Design review of the part built by this model. Coordinates are the model's own, in mm. A direction names the side the tool comes from. Coordinates: 2 decimals unless noted, no trailing zeros. Loops run counter-clockwise (first coordinate to the right, second up) from the corner with the lowest first, then second, coordinate; pieces in that order, holes last. Notation, with made-up numbers: M 51,63 L 84,63 A26 ccw 84,99 Z; hole C 2,17.25 d7. An arc over 180 degrees is marked long. Write item = value, one per line. Start each with the question number.
from build123d import *

# Parameters (mm, degrees)
F0_R     = 9.75
F0_R_2   = 4
F1_DEPTH = 3.9
F0_R_3   = 16
F2_DEPTH = 6.9
F3_R     = 8.2
F3_R_2   = 6.8
F4_DEPTH = 2.1
F3_R_3   = 4
F5_DEPTH = 1.3
F6_R     = 2


with BuildPart() as f1:
    # F0 (on Front) → F1 (new body)
    with BuildSketch(Plane.XZ):
        Circle(F0_R)
        Circle(F0_R_2, mode=Mode.SUBTRACT)
    extrude(amount=F1_DEPTH)

    # F0 (on Front) → F2 (join)
    with BuildSketch(Plane.XZ):
        Circle(F0_R_3)
        Circle(F0_R, mode=Mode.SUBTRACT)
    extrude(amount=F2_DEPTH)

    # F3 (on Front) → F4 (join)
    with BuildSketch(Plane.XZ):
        Circle(F3_R)
        Circle(F3_R_2, mode=Mode.SUBTRACT)
    extrude(amount=-F4_DEPTH)

    # F3 (on Front) → F5 (join)
    with BuildSketch(Plane.XZ):
        Circle(F3_R_2)
        Circle(F3_R_3, mode=Mode.SUBTRACT)
    extrude(amount=-F5_DEPTH)

    # F6
    f6_edges = [f1.edges().sort_by_distance(p)[0] for p in [
        (-16, -6.9, 0),
        (-16, 0, 0),
    ]]
    fillet(f6_edges, radius=F6_R)


solid = f1.part
Q1. To check wall thickness, follow line 1 (Z direction, x = 0, y = 1.6); line 2 (Y direction, x = 7, z = -8.5); line 3 (Z direction, x = 0, y = -1.45). State the ranges of each line that lie inside material, in increasing order. Write a range as from..to.
Q2. Mouldability with a two-part tool opening along Z and no side actions: class faces 1 (the face through (-3.47, -3.43, -15.62)), 2 (the face through (4.2, -3.9, 0.1)), 3 (the face through (6, 0, -6)) as released by +Z, released by -Z, zero draft, split by the parting line, or undercut.
Q3. Add section D-D on y = -0.5. State the section outline as (x, z) points.
Q4. Add section B-B on x = 0. State the section outline as (y, z) points.
Q5. Add section C-C on y = -3.25. State the section outline as (x, z) points, plus the area to 3 significant figures.
Q6. For faces 4 (the face through (3, 1.3, -3)), 5 (the face through (3, -6.9, 10)), 6 (the face through (-1.269, -5.379, 9.667)), list the 3-axis set-ups (+Z, -Z, +X, -X, +Y, -Y) from which the entire face can be reached by the end or side of a thin tool; tool diameter is ignored.
Q7. Add section A-A on z = 0. State the section outline as (x, y) points, plus the area to 3 significant figures.
Q8. Clearance check with flat-ended pins moving along their axes: P1, Ø3, axis at x = -1, z = 12, coming from the +Y side; P2, Ø2, axis at x = -4, y = -3, coming from the +Z side; P3, Ø3, axis at x = -5.5, z = -4.5, coming from the -Y side. State where each tip first meets the part, or that it passes through.
Values follow:
q1.line_1 = -8.2..-6.8, 6.8..8.2
q1.line_2 = -6.9..0
q1.line_3 = -15.92..-4, 4..15.92
q2.face_1 = split by the parting line
q2.face_2 = undercut
q2.face_3 = zero draft
q3.outline = C 0,0 d30.65; hole C 0,0 d8
q4.outline = M -6.9,-14 A2 ccw -4.9,-16 L -2,-16 A2 ccw 0,-14 L 0,-8.2 L 2.1,-8.2 L 2.1,-6.8 L 1.3,-6.8 L 1.3,-4 L -3.9,-4 L -3.9,-9.75 L -6.9,-9.75 Z; M -6.9,9.75 L -3.9,9.75 L -3.9,4 L 1.3,4 L 1.3,6.8 L 2.1,6.8 L 2.1,8.2 L 0,8.2 L 0,14 A2 ccw -2,16 L -4.9,16 A2 ccw -6.9,14 Z
q5.outline = C 0,0 d32; hole C 0,0 d8
q5.area = 754 mm2
q6.face_4 = +Y
q6.face_5 = +Z, -Z, +X, -X, -Y
q6.face_6 = -Y
q7.outline = M -16,-4.9 A2 ccw -14,-6.9 L -9.75,-6.9 L -9.75,-3.9 L -4,-3.9 L -4,1.3 L -6.8,1.3 L -6.8,2.1 L -8.2,2.1 L -8.2,0 L -14,0 A2 ccw -16,-2 Z; M 4,-3.9 L 9.75,-3.9 L 9.75,-6.9 L 14,-6.9 A2 ccw 16,-4.9 L 16,-2 A2 ccw 14,0 L 8.2,0 L 8.2,2.1 L 6.8,2.1 L 6.8,1.3 L 4,1.3 Z
q7.area = 141 mm2
q8.P1 = 0
q8.P2 = 15.72
q8.P3 = -3.9
